Geometry: see drawing. Coordinates: mm, zero at the bounding-box minimum. Give positions to 0.01 mm unless a question says otherwise; leave off trailing zeros. Order: outer loops, then holes, each group sorted by start corner. A loop starts at its lowest first (then second) coordinate and runs counter-clockwise, first axis right, second up. Notation, with made-up numbers: M 46,30 L 102,30 A19 cw 102,45 Z; hole C 67,-9.5 d5. An arc over 180 degrees is marked long. Answer as a JSON object with one key per item and string values. Group by question number.
1. Material intervals for L1, parallel to Z at x = 124, y = 0.4 (1 decimal); L2, parallel to X at y = 1.5, z = 8.5 (1 decimal); L3, parallel to Z at x = 95.5, y = 0.1, sorted ascending. Write a range as [from, to].
2. Section query B-B (y = 0.5). Output: boundary loops of the cut face in (x, z) (1 decimal), plus the area to 3 significant figures.
3. Section query A-A (x = 70.5). Output: boundary loops of the cut face in (y, z), plus the area to 3 significant figures.
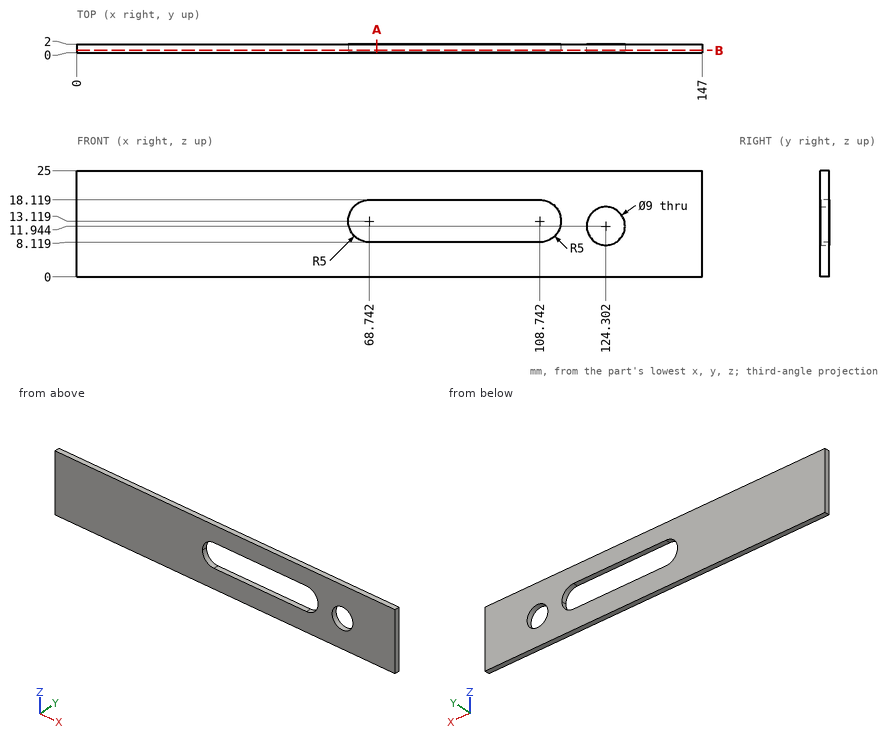
Answer sheet:
{
 "1": {"L1": "[0, 7.5], [16.4, 25]", "L2": "[0, 66.8], [110.7, 121.4], [127.2, 147]", "L3": "[0, 8.12], [18.12, 25]"},
 "2": {"outline": "M 0,0 L 147,0 L 147,25 L 0,25 Z; hole M 68.7,8.1 L 108.7,8.1 A5 ccw 108.7,18.1 L 68.7,18.1 A5 ccw Z; hole C 124.3,11.9 d9", "area": "3,130 mm^2"},
 "3": {"outline": "M 0,0 L 2,0 L 2,8.12 L 0,8.12 Z; M 0,18.12 L 2,18.12 L 2,25 L 0,25 Z", "area": "30.0 mm^2"}
}
